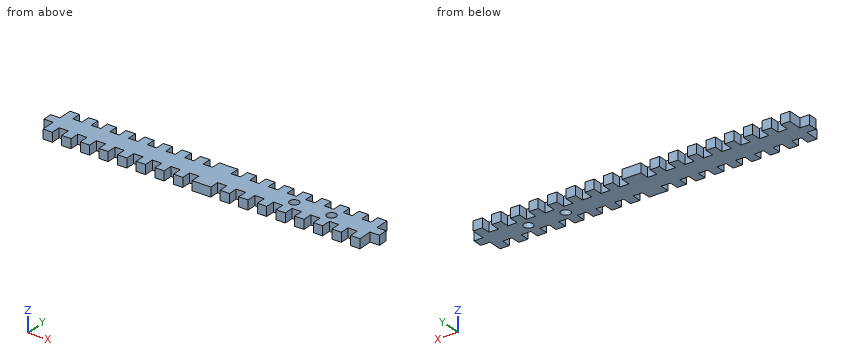
```python
from build123d import *

# Parameters (mm, degrees)
SKETCH2_R           = 3.175
BOSS_EXTRUDE1_DEPTH = 6.35


with BuildPart() as part:
    # Sketch2 → Boss-Extrude1 (new body)
    with BuildSketch(Plane.XY):
        Polygon((-107.95, 12.7), (-101.6, 12.7), (-101.6, 6.35), (-95.25, 6.35), (-95.25, 12.7), (-88.9, 12.7), (-88.9, 6.35), (-82.55, 6.35), (-82.55, 12.7), (-76.2, 12.7), (-76.2, 6.35), (-69.85, 6.35), (-69.85, 12.7), (-63.5, 12.7), (-63.5, 6.35), (-57.15, 6.35), (-57.15, 12.7), (-50.8, 12.7), (-50.8, 6.35), (-44.45, 6.35), (-44.45, 12.7), (-38.1, 12.7), (-38.1, 6.35), (-31.75, 6.35), (-31.75, 12.7), (-25.4, 12.7), (-25.4, 6.35), (-19.05, 6.35), (-19.05, 12.7), (-12.7, 12.7), (-12.7, 6.35), (-6.35, 6.35), (-6.35, 12.7), (6.35, 12.7), (6.35, 6.35), (12.7, 6.35), (12.7, 12.7), (19.05, 12.7), (19.05, 6.35), (25.4, 6.35), (25.4, 12.7), (31.75, 12.7), (31.75, 6.35), (38.1, 6.35), (38.1, 12.7), (44.45, 12.7), (44.45, 6.35), (50.8, 6.35), (50.8, 12.7), (57.15, 12.7), (57.15, 6.35), (63.5, 6.35), (63.5, 12.7), (69.85, 12.7), (69.85, 6.35), (76.2, 6.35), (76.2, 12.7), (82.55, 12.7), (82.55, 6.35), (88.9, 6.35), (88.9, 12.7), (95.25, 12.7), (95.25, 6.35), (101.6, 6.35), (101.6, 12.7), (107.95, 12.7), (107.95, 3.175), (114.3, 3.175), (114.3, -3.175), (107.95, -3.175), (107.95, -12.7), (101.6, -12.7), (101.6, -6.35), (95.25, -6.35), (95.25, -12.7), (88.9, -12.7), (88.9, -6.35), (82.55, -6.35), (82.55, -12.7), (76.2, -12.7), (76.2, -6.35), (69.85, -6.35), (69.85, -12.7), (63.5, -12.7), (63.5, -6.35), (57.15, -6.35), (57.15, -12.7), (50.8, -12.7), (50.8, -6.35), (44.45, -6.35), (44.45, -12.7), (38.1, -12.7), (38.1, -6.35), (31.75, -6.35), (31.75, -12.7), (25.4, -12.7), (25.4, -6.35), (19.05, -6.35), (19.05, -12.7), (12.7, -12.7), (12.7, -6.35), (6.35, -6.35), (6.35, -12.7), (-6.35, -12.7), (-6.35, -6.35), (-12.7, -6.35), (-12.7, -12.7), (-19.05, -12.7), (-19.05, -6.35), (-25.4, -6.35), (-25.4, -12.7), (-31.75, -12.7), (-31.75, -6.35), (-38.1, -6.35), (-38.1, -12.7), (-44.45, -12.7), (-44.45, -6.35), (-50.8, -6.35), (-50.8, -12.7), (-57.15, -12.7), (-57.15, -6.35), (-63.5, -6.35), (-63.5, -12.7), (-69.85, -12.7), (-69.85, -6.35), (-76.2, -6.35), (-76.2, -12.7), (-82.55, -12.7), (-82.55, -6.35), (-88.9, -6.35), (-88.9, -12.7), (-95.25, -12.7), (-95.25, -6.35), (-101.6, -6.35), (-101.6, -12.7), (-107.95, -12.7), (-107.95, -3.175), (-114.3, -3.175), (-114.3, 3.175), (-107.95, 3.175), align=None)
        with Locations((79.375, 0)):
            Circle(SKETCH2_R, mode=Mode.SUBTRACT)
        with Locations((53.975, 0)):
            Circle(SKETCH2_R, mode=Mode.SUBTRACT)
    extrude(amount=BOSS_EXTRUDE1_DEPTH)


solid = part.part
```
CAD build for the part. Positions are in the model's coordinates, mm. Round coordinates to 2 decimals unless told otherwise and drop trailing zeros. Use CSV: the item, a comma, the result in double quotes. Start each with the question number.
1) Saw through at B-B (y = -10). Count the separate pieces of the cut face and the enclosed holes in it, and give its area (3 significant figures).
2) Pin check, flat tips, straight feed: pin 1 Ø3 at (x, z) = (-112.5, 3.5) entering from -Y (3 decimals); pin 2 Ø1.9 at (y, z) = (-10, 4.5) entering from -X; pin 3 Ø1.9 at (y, z) = (-11, 3) entering from +X. Stop position of each tip, or through.
3) Wall check: L1, parallel to X at y = 0.5, z = 0.5; L2, parallel to X at y = 1.5, z = 4; L3, parallel to Y at x = 58.5, z = 2.5. Give the ranges that are in metal, low to high. Write a range as [from, to].
Values follow:
1,separate pieces,"17"
1,enclosed holes,"0"
1,area,"726 mm2"
2,pin 1,"stops at y = -3.175"
2,pin 2,"stops at x = -107.95"
2,pin 3,"stops at x = 107.95"
3,L1,"x = [-114.3, 50.84], [57.11, 76.24], [82.51, 114.3]"
3,L2,"x = [-114.3, 51.18], [56.77, 76.58], [82.17, 114.3]"
3,L3,"y = [-6.35, 6.35]"
